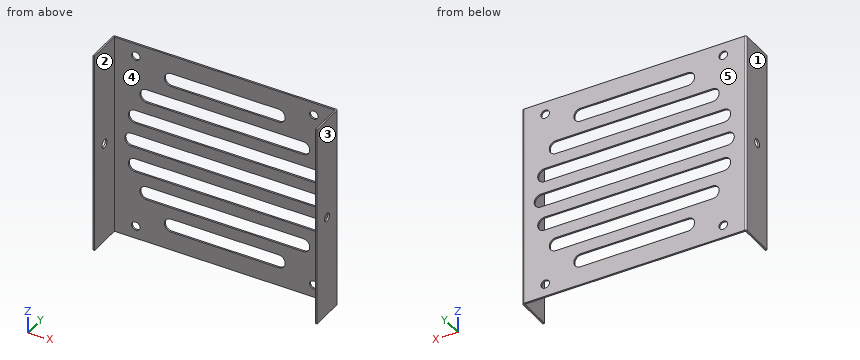
from build123d import *

# Parameters (mm, degrees)
SKETCH1_W               = 130
SKETCH1_H               = 120
SKETCH1_R               = 2.5
BOSS_EXTRUDE1_DEPTH     = 1
EDGE_FLANGE1_DEPTH      = 120
CUT_EXTRUDE1_DEPTH      = 92.48338647
CUT_EXTRUDE1_DEPTH_BACK = 92.48338647
SKETCH10_R              = 2.5


# Sheet-metal steps are written as plain solids
with BuildPart() as part:
    # Sketch1 → Boss-Extrude1 (new body)
    with BuildSketch(Plane(origin=(0, 0, 0), x_dir=(1, 0, 0), z_dir=(0, 1, 0))):
        Rectangle(SKETCH1_W, SKETCH1_H)
        with Locations(Location((-52.5, 52.5, 0), (0, 0, 270))):
            Circle(SKETCH1_R, mode=Mode.SUBTRACT)
        with Locations(Location((52.5, 52.5, 0), (0, 0, 90))):
            Circle(SKETCH1_R, mode=Mode.SUBTRACT)
        with Locations(Location((52.5, -52.5, 0), (0, 0, 270))):
            Circle(SKETCH1_R, mode=Mode.SUBTRACT)
        with Locations(Location((-52.5, -52.5, 0), (0, 0, 90))):
            Circle(SKETCH1_R, mode=Mode.SUBTRACT)
        with BuildLine():
            Line((-31.622776602, 49), (31.622776602, 49))
            ThreePointArc((31.622776602, 49), (35.622776602, 45), (31.622776602, 41))
            Line((31.622776602, 41), (-31.622776602, 41))
            ThreePointArc((-31.622776602, 41), (-35.622776602, 45), (-31.622776602, 49))
        make_face(mode=Mode.SUBTRACT)
        with BuildLine():
            Line((-46.097722286, 34), (46.097722286, 34))
            ThreePointArc((46.097722286, 34), (50.097722286, 30), (46.097722286, 26))
            Line((46.097722286, 26), (-46.097722286, 26))
            ThreePointArc((-46.097722286, 26), (-50.097722286, 30), (-46.097722286, 34))
        make_face(mode=Mode.SUBTRACT)
        with BuildLine():
            Line((-52.915026221, 19), (52.915026221, 19))
            ThreePointArc((52.915026221, 19), (56.915026221, 15), (52.915026221, 11))
            Line((52.915026221, 11), (-52.915026221, 11))
            ThreePointArc((-52.915026221, 11), (-56.915026221, 15), (-52.915026221, 19))
        make_face(mode=Mode.SUBTRACT)
        with BuildLine():
            Line((-55, 4), (55, 4))
            ThreePointArc((55, 4), (59, 0), (55, -4))
            Line((55, -4), (-55, -4))
            ThreePointArc((-55, -4), (-59, 0), (-55, 4))
        make_face(mode=Mode.SUBTRACT)
        with BuildLine():
            Line((-52.915026221, -19), (52.915026221, -19))
            ThreePointArc((52.915026221, -19), (56.915026221, -15), (52.915026221, -11))
            Line((52.915026221, -11), (-52.915026221, -11))
            ThreePointArc((-52.915026221, -11), (-56.915026221, -15), (-52.915026221, -19))
        make_face(mode=Mode.SUBTRACT)
        with BuildLine():
            Line((-46.097722286, -34), (46.097722286, -34))
            ThreePointArc((46.097722286, -34), (50.097722286, -30), (46.097722286, -26))
            Line((46.097722286, -26), (-46.097722286, -26))
            ThreePointArc((-46.097722286, -26), (-50.097722286, -30), (-46.097722286, -34))
        make_face(mode=Mode.SUBTRACT)
        with BuildLine():
            Line((-31.622776602, -49), (31.622776602, -49))
            ThreePointArc((31.622776602, -49), (35.622776602, -45), (31.622776602, -41))
            Line((31.622776602, -41), (-31.622776602, -41))
            ThreePointArc((-31.622776602, -41), (-35.622776602, -45), (-31.622776602, -49))
        make_face(mode=Mode.SUBTRACT)
    extrude(amount=BOSS_EXTRUDE1_DEPTH)

    # Edge-Flange1 section (across the edge) → Edge-Flange1 (add)
    with BuildSketch(Plane(origin=(-65.1, 0, 60), x_dir=(1, 0, 0), z_dir=(0, 0, -1))):
        with BuildLine():
            Line((-1, 0.1), (-1, 20))
            Line((-1, 20), (0, 20))
            Line((0, 20), (0, 0.1))
            ThreePointArc((0, 0.1), (0.029289322, 0.029289322), (0.1, 0))
            Line((0.1, 0), (0.1, -1))
            ThreePointArc((0.1, -1), (-0.677817459, -0.677817459), (-1, 0.1))
        make_face()
    edge_flange1 = extrude(amount=EDGE_FLANGE1_DEPTH)

    # Mirror1: Edge-Flange1 across plane
    add(edge_flange1.mirror(Plane(origin=(0, 0, 0), x_dir=(0, 0, 1), z_dir=(1, 0, 0))))

    # Sketch10 → Cut-Extrude1 (cut, two sides: drawn at the far end of the back side and taken through both)
    with BuildSketch(Plane(origin=(0, 0, 0), x_dir=(0, 0, -1), z_dir=(1, 0, 0)).offset(-CUT_EXTRUDE1_DEPTH_BACK)):
        with Locations((0, -10)):
            Circle(SKETCH10_R)
    extrude(amount=CUT_EXTRUDE1_DEPTH + CUT_EXTRUDE1_DEPTH_BACK, mode=Mode.SUBTRACT)


solid = part.part
Verification items for the finished model (mm, model axes). Face numbers are marked on the shaded views. A direction names the side the tool comes from. Coordinates: 2 decimals unless noted, no trailing zeros. Write each loop counter-clockwise with the first axis right and the second up, starting at its lowest first coordinate (ties: lowest second). Pieces come first, ordered by that corner, then holes. Notation, with made-up numbers: M -23,72.5 L -17,72.5 A21 ccw -17,93.5 Z; hole C 44.25,88 d3. An arc over 180 degrees is marked long. Use a Markdown table: item, result.
Q1. Sectioned sample at B-B, the plane z = 45. Record the boundary of the cut face in (x, y).
Reply:
| item | result |
|---|---|
| outline | M -66.1,-20 L -65.1,-20 L -65.1,-0.1 A0.1 cw -65,0 L -35.62,0 L -35.62,1 L -65,1 A1.1 ccw -66.1,-0.1 Z; M 35.62,0 L 65,0 A0.1 cw 65.1,-0.1 L 65.1,-20 L 66.1,-20 L 66.1,-0.1 A1.1 ccw 65,1 L 35.62,1 Z |
Q2. Go/stop test with a flat-tipped pin: P1, Ø12, axis at x = 31.5, z = 18.5, coming from the -Y side. Record where the tip stops, or that it passes through.
Reply:
| item | result |
|---|---|
| P1 | stops at y = 0 |
Q3. Thickness scan on line 1 (Y direction, x = -65.25, z = 0); line 2 (X direction, y = -14.5, z = -23.5); line 3 (X direction, y = 0.3, z = -52.5). Record the ranges inside material, lowest first.
Reply:
| item | result |
|---|---|
| line 1 | y = -20 to -12.5, -7.5 to 0.97 |
| line 2 | x = -66.1 to -65.1, 65.1 to 66.1 |
| line 3 | x = -66.02 to -55, -50 to 50, 55 to 66.02 |
Q4. Sectioned sample at A-A, the plane y = -5.75. Record the boundary of the cut face in (x, z).
Reply:
| item | result |
|---|---|
| outline | M -66.1,-60 L -65.1,-60 L -65.1,60 L -66.1,60 Z; M 65.1,-60 L 66.1,-60 L 66.1,60 L 65.1,60 Z |
Q5. Sectioned sample at C-C, the plane x = 11.5. Count the separate pieces of the cut face and the enclosed holes in it, plus the area to 3 significant figures.
Reply:
| item | result |
|---|---|
| separate pieces | 8 |
| enclosed holes | 0 |
| area | 64.0 mm² |
Q6. Sectioned sample at D-D, the plane z = -6. Record the boundary of the cut face in (x, y).
Reply:
| item | result |
|---|---|
| outline | M -66.1,-20 L -65.1,-20 L -65.1,-0.1 A0.1 cw -65,0 L 65,0 A0.1 cw 65.1,-0.1 L 65.1,-20 L 66.1,-20 L 66.1,-0.1 A1.1 ccw 65,1 L -65,1 A1.1 ccw -66.1,-0.1 Z |
Q7. Set-up check for the marked faces 1 and 2: record each of +Z, -Z, +X, -X, +Y, -Y from which the full face is reachable in a straight line by a thin tool's end or side.
Reply:
| item | result |
|---|---|
| face 1 | +Z, -Z, -X, +Y, -Y |
| face 2 | +Z, -Z, -Y |
Q8. Draft check along X on the marked faces 3, 4 and 5. Enter one of: +X half, -X half, draft (parallel to the pull), parting line (faces both ways), or undercut.
Reply:
| item | result |
|---|---|
| face 3 | +X half |
| face 4 | undercut |
| face 5 | draft |
